Here's how the part is built. I have some questions about the finished solid (model axes, mm). A direction names the side the tool comes from. Round coordinates to 2 decimals unless told otherwise and drop trailing zeros. Loops run counter-clockwise (first coordinate to the right, second up) from the corner with the lowest first, then second, coordinate; pieces in that order, holes last. Notation, with made-up numbers: M 43,47.5 L 65,47.5 A29 cw 65,83.5 Z; hole C 89,40.25 d1. An arc over 180 degrees is marked long. Use a Markdown table: item, result.
from build123d import *

# Parameters (mm, degrees)
F1_DEPTH = 98
F2_W     = 26
F2_H     = 10
F3_DEPTH = 2
F4_W     = 22
F4_H     = 2
F5_DEPTH = 8


with BuildPart() as f1:
    # F0 (on Top) → F1 (new body)
    with BuildSketch(Plane.XY):
        Polygon((2, 0), (0, 0), (0, -10), (26, -10), (26, 0), (24, 0), (24, -8), (2, -8), align=None)
    extrude(amount=F1_DEPTH)

    # F2 (on face) → F3 (join)
    with BuildSketch(Plane.XY.offset(98)):
        with Locations((13, -5)):
            Rectangle(F2_W, F2_H)
    extrude(amount=F3_DEPTH)

    # F4 (on face) → F5 (join, through all)
    with BuildSketch(Plane(origin=(0, -8, 0), x_dir=(-1, 0, 0), z_dir=(0, 1, 0))):
        with Locations((-13, 65)):
            Rectangle(F4_W, F4_H)
        with Locations((-13, 31)):
            Rectangle(F4_W, F4_H)
    extrude(amount=F5_DEPTH)


solid = f1.part
1. Which directions (+Z, -Z, +X, -X, +Y, -Y) give clear straight access to the entire face, cutting with the end or side of a thin tool? Please do faces 1 (the face through (24, -4, 15)), 2 (the face through (13, -4, 98)), 3 (the face through (0, -5, 49)).
Answer sheet:
| item | result |
|---|---|
| face 1 | -Z, +Y |
| face 2 | +Y |
| face 3 | +Z, -Z, -X, +Y, -Y |
2. For pin 1 Ø1 at (x, z) = (17, 34) entering from +Y; pin 2 Ø2.5 at (x, y) = (17, -3) entering from -Z, each with a flat end and sliding along its axis, tell me the tip position at first contact or that it passes through.
Answer sheet:
| item | result |
|---|---|
| pin 1 | y = -8 |
| pin 2 | z = 30 |
3. Imagine slicing it at B-B, the plane z = 8. Write out the boundary of the cut face in (x, y), then the cut area to 3 significant figures.
Answer sheet:
| item | result |
|---|---|
| outline | M 0,-10 L 26,-10 L 26,0 L 24,0 L 24,-8 L 2,-8 L 2,0 L 0,0 Z |
| area | 84.0 mm2 |
4. We'd pull the mould along X, two halves only. Please class faces 4 (the face through (26, -5, 49)), 5 (the face through (13, -8, 15)), 6 (the face through (12.8, -8.3, 0)), 7 (the face through (24, -4, 82)): +X half, -X half, draft (parallel to the pull), parting line (faces both ways), or undercut.
Answer sheet:
| item | result |
|---|---|
| face 4 | +X half |
| face 5 | undercut |
| face 6 | draft |
| face 7 | undercut |
5. I need wall thicknesses on probe 1 along Z at (x, y) = (9, -2); probe 2 along X at (y, z) = (-5, 63); probe 3 along Y at (x, z) = (19.75, 78). Which ranges of each line are inside material? Lowest first, please. Write a range as from..to.
Answer sheet:
| item | result |
|---|---|
| probe 1 | 30..32, 64..66, 98..100 |
| probe 2 | 0..2, 24..26 |
| probe 3 | -10..-8 |
6. Imagine slicing it at A-A, the plane y = -3. Write out the boundary of the cut face in (x, z).
Answer sheet:
| item | result |
|---|---|
| outline | M 0,0 L 2,0 L 2,30 L 24,30 L 24,0 L 26,0 L 26,100 L 0,100 Z; hole M 2,32 L 24,32 L 24,64 L 2,64 Z; hole M 2,66 L 24,66 L 24,98 L 2,98 Z |
7. Imagine slicing it at C-C, the plane x = 23. Write out the boundary of the cut face in (y, z).
Answer sheet:
| item | result |
|---|---|
| outline | M -10,0 L -8,0 L -8,30 L 0,30 L 0,32 L -8,32 L -8,64 L 0,64 L 0,66 L -8,66 L -8,98 L 0,98 L 0,100 L -10,100 Z |
